Input: part model. Units: mm. Frame: model coordinates. Face numbers are marked on the shaded views. A direction names the side the tool comes from. Give positions to 0.01 mm unless a question says otherwise; leave off trailing zeros. Order: outer loops, then holes, each group sorted by start corner. A loop starts at its lowest first (then second) coordinate and runs counter-clockwise, first axis right, second up. Notation, with made-up numbers: (20, 76.25) -> (73, 76.25) arc R31 cw to (73, 104.25) -> close; hole circle Ø7 at (70, 37). An arc over 180 degrees is marked (long way). Use a Markdown table: item, result. Add a question column.
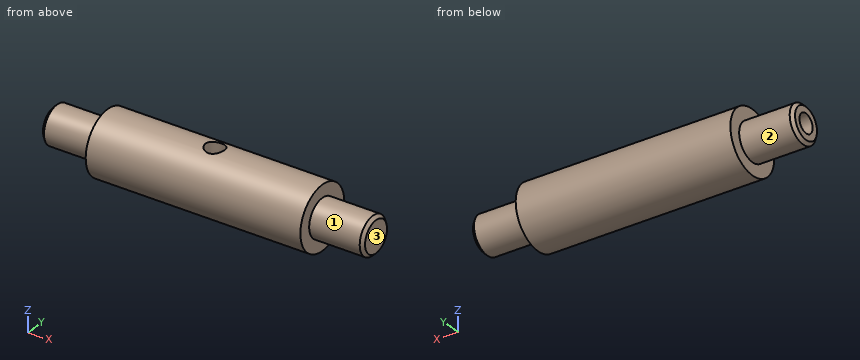
from build123d import *

# Parameters (mm, degrees)
F2_SIZE  = 1
F3_R     = 3
F4_DEPTH = 57
F5_R     = 3
F6_DEPTH = 32


with BuildPart() as f1:
    # F0 (on Front) → F1 (revolve)
    with BuildSketch(Plane.XZ):
        Polygon((-51, 6), (-51, 0), (51, 0), (51, 6), (34, 6), (34, 10), (-34, 10), (-34, 6), align=None)
    revolve(axis=Axis((0, 0, 0), (1, 0, 0)))

    # F2
    f2_edges = [f1.edges().sort_by_distance(p)[0] for p in [
        (51, 0, -6),
        (-51, 0, -6),
    ]]
    chamfer(f2_edges, length=F2_SIZE)

    # F3 (on face) → F4 (cut)
    with BuildSketch(Plane(origin=(-51, 0, 0), x_dir=(0, -1, 0), z_dir=(-1, 0, 0))):
        Circle(F3_R)
    extrude(amount=-F4_DEPTH, mode=Mode.SUBTRACT)

    # F5 (on Top) → F6 (cut)
    with BuildSketch(Plane.XY):
        Circle(F5_R)
    extrude(amount=F6_DEPTH, mode=Mode.SUBTRACT)


solid = f1.part
Q1. First-contact query: pin 1 (1.5 mm diameter, centred on x = -20.5, z = 4, fed in from -Y); pin 2 (1 mm diameter, centred on x = 25, z = -1.5, fed in from +Y); pin 3 (8 mm diameter, centred on x = -5, z = 1.5, fed in from +Y); pin 4 (6 mm diameter, centred on x = 38, y = -7.5, fed in from -Z). Flat tips, straight axial feed; report the tip coordinate or a pass-through.
Q2. Access query for the marked faces 1, 2 and 3. Directions: +Z, -Z, +X, -X, +Y, -Y. A direction counts if a zero-diameter tool reaches every point of the face in a straight line with its end or side. Return the directions, or none.
Q3. Section query B-B (z = 8). Return loops of the section in (x, y), plus the area to 3 significant figures.
Q4. Section query A-A (y = 0). Return loops of the section in (x, z), plus the area to 3 significant figures.
Q5. Section query C-C (x = 5). Return loops of the section in (y, z).
Q6. Section query D-D (y = 8). Return loops of the section in (x, z), plus the area to 3 significant figures.
Q7. Ray query, line 1 (X direction, y = 0, z = 4.25); line 2 (Y direction, x = -26, z = 0); line 3 (X direction, y = 0, z = 6.25). Return the intervals inside material, ascending.
Solution:
| question | item | result |
|---|---|---|
| 1 | pin 1 | stops at y = -9.46 |
| 1 | pin 2 | stops at y = 9.95 |
| 1 | pin 3 | stops at y = 10 |
| 1 | pin 4 | stops at z = -3.97 |
| 2 | face 1 | +X |
| 2 | face 2 | -X |
| 2 | face 3 | +Z, -Z, +X, +Y, -Y |
| 3 | outline | (-34, -6) -> (34, -6) -> (34, 6) -> (-34, 6) -> close; hole circle Ø6 at (0, 0) |
| 3 | area | 788 mm² |
| 4 | outline | (-51, -5) -> (-50, -6) -> (-34, -6) -> (-34, -10) -> (34, -10) -> (34, -6) -> (50, -6) -> (51, -5) -> (51, 5) -> (50, 6) -> (34, 6) -> (34, 10) -> (3, 10) -> (3, 3) -> (6, 3) -> (6, -3) -> (-51, -3) -> close; (-51, 3) -> (-3, 3) -> (-3, 10) -> (-34, 10) -> (-34, 6) -> (-50, 6) -> (-51, 5) -> close |
| 4 | area | 1,380 mm² |
| 5 | outline | circle Ø20 at (0, 0); hole circle Ø6 at (0, 0) |
| 6 | outline | (-34, -6) -> (34, -6) -> (34, 6) -> (-34, 6) -> close |
| 6 | area | 816 mm² |
| 7 | line 1 | x = -51 to -3, 3 to 51 |
| 7 | line 2 | y = -10 to -3, 3 to 10 |
| 7 | line 3 | x = -34 to -3, 3 to 34 |
